The model under review builds one solid part; all positions refer to its coordinate system, in mm. A direction names the side the tool comes from. Give positions to 0.01 mm unless a question says otherwise; leave off trailing zeros. Loops run counter-clockwise (first coordinate to the right, second up) from the corner with the lowest first, then second, coordinate; pieces in that order, holes last. Notation, with made-up numbers: M 80.5,14 L 135.5,14 A20 cw 135.5,31 Z; hole C 9,27.25 d4. An arc over 180 degrees is marked long. One line per item, written item: value. Start each with the question number.
Q1. We need section C-C on y = 15.25. Write out the cut boundary in (x, z), plus the area to 3 significant figures.
Q2. For faces 1 (the face through (-4, 7, 0)), 2 (the face through (1.3, 18.1, -1.75)), list the 3-axis set-ups (+Z, -Z, +X, -X, +Y, -Y) from which the entire face can be reached by the end or side of a thin tool; tool diameter is ignored.
Q3. We need section B-B on y = 9.75. Write out the cut boundary in (x, z).
Q4. We need section A-A on z = -3. Write out the cut boundary in (x, y).
Q5. For pin 1 (1 mm diameter, centred on x = 1.5, z = -2.5, fed in from +Y); pin 2 (5 mm diameter, centred on x = 6, z = -3.5, fed in from +Y); pin 3 (1 mm diameter, centred on x = 1, y = 17, fed in from +Z); pin 4 (1 mm diameter, centred on x = 4, y = 16.5, fed in from -Z), all flat-tipped, find the tip position at first contact; note any pin that passes through.
Q6. To check wall thickness, follow line 1 along Z through (x, y) = (-4.25, 12.75); line 2 along Z through (x, y) = (4.5, 2); line 3 along X through (y, z) = (4.5, 2). State the ranges of each line that lie inside material, in increasing order. Write a range as from..to.
Q7. Mouldability with a two-part tool opening along X and no side actions: class faces 3 (the face through (0, 4, 4.7)), 4 (the face through (-2, 7, -7.5)), 5 (the face through (3, 18, 0)) as released by +X, released by -X, zero draft, split by the parting line, or undercut.
```python
from build123d import *
from build123d.topology import SkipClean

# Parameters (mm, degrees)
SKETCH_1_W               = 15
SKETCH_1_H               = 15
EXTRUDE_1_DEPTH          = 15
CUT_EXTRUDE_1_DEPTH      = 9
SKETCH_4_W               = 3
SKETCH_4_H               = 6.5
EXTRUDE_2_DEPTH          = 0.5
EXTRUDE_3_DEPTH          = 2.2
EXTRUDE_3_DEPTH_BACK     = 0.5
SKETCH_6_R               = 2
SKETCH_7_W               = 6
SKETCH_7_H               = 3.5
EXTRUDE_4_DEPTH          = 1.3
EXTRUDE_START            = 0.8
SKETCH_8_R               = 2
EXTRUDE_5_DEPTH          = 0.8
CHAMFER_1_SIZE           = 0.5
CUT_EXTRUDE_2_DEPTH      = 2
CUT_EXTRUDE_2_DEPTH_BACK = 2
PATTERN_CIRCULAR_1_COUNT = 4
CUT_EXTRUDE_3_DEPTH      = 13.6


with BuildPart() as part:
    # 草图1 → 凸台-拉伸1 (new body)
    with BuildSketch(Plane(origin=(0, 0, 0), x_dir=(1, 0, 0), z_dir=(0, 1, 0))):
        Rectangle(SKETCH_1_W, SKETCH_1_H)
    extrude(amount=EXTRUDE_1_DEPTH)

    # 草图2 → 切除-拉伸1 (cut)
    with BuildSketch(Plane.XZ):
        with BuildLine():
            Line((1.5, 7.5), (-1.5, 7.5))
            Line((-1.5, 7.5), (-1.5, 6.822875656))
            ThreePointArc((-1.5, 6.822875656), (-1.780042303, 6.411838473), (-1.95, 5.944409721))
            Line((-1.95, 5.944409721), (-1.95, 4.7))
            Line((-1.95, 4.7), (1.95, 4.7))
            Line((1.95, 4.7), (1.95, 5.944409721))
            ThreePointArc((1.95, 5.944409721), (1.780042303, 6.411838473), (1.5, 6.822875656))
            Line((1.5, 6.822875656), (1.5, 7.5))
        make_face()
    cut_extrude_1 = extrude(amount=-CUT_EXTRUDE_1_DEPTH, mode=Mode.SUBTRACT)

    # 草图4 → 凸台-拉伸2 (add)
    with BuildSketch(Plane(origin=(0, 15, 0), x_dir=(1, 0, 0), z_dir=(0, 1, 0))):
        Rectangle(SKETCH_4_W, SKETCH_4_H)
    extrude(amount=EXTRUDE_2_DEPTH)

    # 草图6 → 凸台-拉伸3 (add, two sides: drawn at the far end of the back side and taken through both)
    with BuildSketch(Plane(origin=(0, 15.5, 0), x_dir=(1, 0, 0), z_dir=(0, 1, 0)).offset(-EXTRUDE_3_DEPTH_BACK)):
        with Locations(Location((0, 0, 0), (0, 0, 270))):
            Circle(SKETCH_6_R)
    extrude(amount=EXTRUDE_3_DEPTH + EXTRUDE_3_DEPTH_BACK)

    # 草图7 → 凸台-拉伸4 (add)
    with BuildSketch(Plane(origin=(0, 17.7, 0), x_dir=(1, 0, 0), z_dir=(0, 1, 0))):
        Rectangle(SKETCH_7_W, SKETCH_7_H)
    extrude(amount=EXTRUDE_4_DEPTH)

    # 草图8 → 凸台-拉伸5 (add)
    with SkipClean():  # the faces are left unmerged after this step: merging them gives an invalid solid
        with BuildSketch(Plane(origin=(0, 17.7, 0), x_dir=(1, 0, 0), z_dir=(0, 1, 0)).offset(EXTRUDE_START)):
            with Locations(Location((0, 0, 0), (0, 0, 298.955024372))):
                Circle(SKETCH_8_R)
        extrude(amount=-EXTRUDE_5_DEPTH)
    add(part.part.scale(1), mode=Mode.REPLACE)  # the faces are merged on a copy

    # 倒角1
    chamfer_1_edges = [part.edges().sort_by_distance(p)[0] for p in [
        (0, 19, -1.75),
        (-3, 19, 0),
        (0, 19, 1.75),
        (3, 19, 0),
    ]]
    chamfer(chamfer_1_edges, length=CHAMFER_1_SIZE - 0.0001)  # a hair under: the kernel refuses the full size

    # 草图9 → 切除-拉伸2 (cut, two sides: drawn at the far end of the back side and taken through both)
    with BuildSketch(Plane(origin=(0, 0, 0), x_dir=(0, 0, -1), z_dir=(1, 0, 0)).offset(-CUT_EXTRUDE_2_DEPTH_BACK)):
        Polygon((-2, 17.7), (-2, 18.5), (-1.75, 18.5), align=None)
        Polygon((1.75, 18.5), (2, 17.7), (2, 18.5), align=None)
    extrude(amount=CUT_EXTRUDE_2_DEPTH + CUT_EXTRUDE_2_DEPTH_BACK, mode=Mode.SUBTRACT)

    # 阵列(圆周)1: 切除-拉伸1 ×4 about axis
    pattern_circular_1_axis = Axis((0, 0, 0), (0, 1, 0))
    for i in range(1, PATTERN_CIRCULAR_1_COUNT):
        add(cut_extrude_1.rotate(pattern_circular_1_axis, i * 360 / PATTERN_CIRCULAR_1_COUNT), mode=Mode.SUBTRACT)

    # 草图10 → 切除-拉伸3 (cut)
    with BuildSketch(Plane.XZ):
        Polygon((6.8, 6.8), (6.8, 5.3), (4, 2.5), (4, -2.5), (6.8, -5.3), (6.8, -6.8), (5.3, -6.8), (2.5, -4), (-2.5, -4), (-5.3, -6.8), (-6.8, -6.8), (-6.8, -5.3), (-4, -2.5), (-4, 2.5), (-6.8, 5.3), (-6.8, 6.8), (-5.3, 6.8), (-2.5, 4), (2.5, 4), (5.3, 6.8), align=None)
    extrude(amount=-CUT_EXTRUDE_3_DEPTH, mode=Mode.SUBTRACT)


solid = part.part
```
Solved:
1. outline: M -1.5,-3.25 L 1.5,-3.25 L 1.5,-1.32 A2 ccw 1.5,1.32 L 1.5,3.25 L -1.5,3.25 L -1.5,1.32 A2 ccw -1.5,-1.32 Z
1. area: 21.3 mm2
2. face 1: -Y
2. face 2: -Z, +Y
3. outline: M -7.5,-7.5 L 7.5,-7.5 L 7.5,7.5 L -7.5,7.5 Z; hole M -6.8,-6.8 L -5.3,-6.8 L -2.5,-4 L 2.5,-4 L 5.3,-6.8 L 6.8,-6.8 L 6.8,-5.3 L 4,-2.5 L 4,2.5 L 6.8,5.3 L 6.8,6.8 L 5.3,6.8 L 2.5,4 L -2.5,4 L -5.3,6.8 L -6.8,6.8 L -6.8,5.3 L -4,2.5 L -4,-2.5 L -6.8,-5.3 Z
4. outline: M -7.5,0 L -4.5,0 L -4.5,13.6 L 4.5,13.6 L 4.5,0 L 7.5,0 L 7.5,15 L 1.5,15 L 1.5,15.5 L -1.5,15.5 L -1.5,15 L -7.5,15 Z
5. pin 1: y = 15.5
5. pin 2: y = 15
5. pin 3: z = 1.94
5. pin 4: through
6. line 1: -7.5..-5.75, -2.75..2.75, 5.75..7.5
6. line 2: -7.5..-6, -3..3, 6..7.5
6. line 3: -7.5..-4, 4..7.5
7. face 3: undercut
7. face 4: zero draft
7. face 5: released by +X
